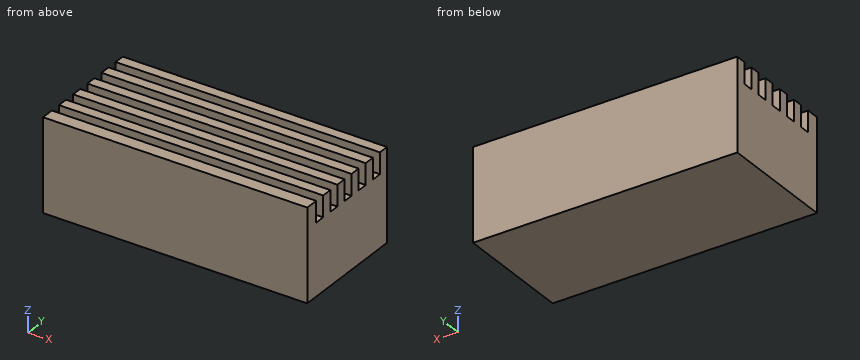
Autodesk Inventor part; units mm, degrees
ref_plane "YZ Plane" through (0, 0, 0) normal (1, 0, 0) x (0, 1, 0)
ref_plane "XZ Plane" through (0, 0, 0) normal (0, 1, 0) x (-1, 0, 0)
ref_plane "XY Plane" through (0, 0, 0) normal (0, 0, 1) x (1, 0, 0)
sketch "Sketch1" plane through (0, 0, 0) normal (0, 0, 1) x (1, 0, 0)
  line L0 (0, 0) -> (63.5, 0)
  line L1 (63.5, 0) -> (63.5, 28.575)
  line L2 (63.5, 28.575) -> (0, 28.575)
  line L3 (0, 28.575) -> (0, 0)
  dimension "d0" = 63.5
  dimension "d1" = 28.575
extrude "Extrusion1" add sketch "Sketch1" along normal blind 22.225
sketch "Sketch2" plane through (0, 0, 22.225) normal (0, 0, 1) x (1, 0, 0)
  line L0 (63.5, 0) -> (63.5, 28.575)
  line L1 (0, 28.575) -> (0, 0)
  line L2 (63.5, 26.035) -> (0, 26.035)
  line L3 (0, 26.035) -> (0, 23.495)
  line L4 (0, 23.495) -> (63.5, 23.495)
  line L5 (63.5, 23.495) -> (63.5, 26.035)
  line L6 (63.5, 28.575) -> (0, 28.575)
  line L7 (63.5, 20.955) -> (0, 20.955)
  line L8 (0, 20.955) -> (0, 18.415)
  line L9 (0, 18.415) -> (63.5, 18.415)
  line L10 (63.5, 18.415) -> (63.5, 20.955)
  line L11 (63.5, 15.875) -> (0, 15.875)
  line L12 (0, 15.875) -> (0, 13.335)
  line L13 (0, 13.335) -> (63.5, 13.335)
  line L14 (63.5, 13.335) -> (63.5, 15.875)
  line L15 (63.5, 10.795) -> (0, 10.795)
  line L16 (0, 10.795) -> (0, 8.255)
  line L17 (0, 8.255) -> (63.5, 8.255)
  line L18 (63.5, 8.255) -> (63.5, 10.795)
  line L19 (63.5, 5.715) -> (0, 5.715)
  line L20 (0, 5.715) -> (0, 3.175)
  line L21 (0, 3.175) -> (63.5, 3.175)
  line L22 (63.5, 3.175) -> (63.5, 5.715)
  dimension "d4" = 2.54
  dimension "d5" = 2.54
  dimension "d8" = 5.08
extrude "Extrusion2" cut sketch "Sketch2" against normal blind 5.08 contours L21 L1 L19 L0 | L17 L1 L15 L0 | L13 L1 L11 L0 | L9 L1 L7 L0 | L4 L1 L2 L0
properties part number "Victor2"
Work out the finished part from the listing and answer in its coordinate system (mm). Coordinates: 2 decimals unless noted, no trailing zeros. Write each loop counter-clockwise with the first axis right and the second up, starting at its lowest first coordinate (ties: lowest second). Pieces come first, ordered by that corner, then holes.
Q1. Find the intervals of material crossed by line 1 (Y direction, x = 53.5, z = 17.5) (3 decimals); line 2 (Z direction, x = 11, y = 9) (3 decimals), in increasing order.
Q2. A cutting plane is placed at A-A, the plane x = 18. Give the vertices of the cut face in (y, z) (3 decimals), then the cut area to 3 significant figures.
Q3. Each of these flat-tipped pins is pushed along its axis until it touches: pin 1 Ø5.5 at (x, z) = (31, 20) entering from -Y; pin 2 Ø1.3 at (x, y) = (22, 20) entering from +Z (3 decimals). Where does it stop, or does it pass through?
Q4. A cutting plane is placed at B-B, the plane y = 24.25. Give the vertices of the cut face in (x, z) (3 decimals), then the cut area to 3 significant figures.
Findings below:
1. line 1: y = 0 to 3.175, 5.715 to 8.255, 10.795 to 13.335, 15.875 to 18.415, 20.955 to 23.495, 26.035 to 28.575
1. line 2: z = 0 to 17.145
2. outline: (0, 0) - (28.575, 0) - (28.575, 22.225) - (26.035, 22.225) - (26.035, 17.145) - (23.495, 17.145) - (23.495, 22.225) - (20.955, 22.225) - (20.955, 17.145) - (18.415, 17.145) - (18.415, 22.225) - (15.875, 22.225) - (15.875, 17.145) - (13.335, 17.145) - (13.335, 22.225) - (10.795, 22.225) - (10.795, 17.145) - (8.255, 17.145) - (8.255, 22.225) - (5.715, 22.225) - (5.715, 17.145) - (3.175, 17.145) - (3.175, 22.225) - (0, 22.225) - close
2. area: 571 mm2
3. pin 1: stops at y = 0
3. pin 2: stops at z = 17.145
4. outline: (0, 0) - (63.5, 0) - (63.5, 17.145) - (0, 17.145) - close
4. area: 1,090 mm2
